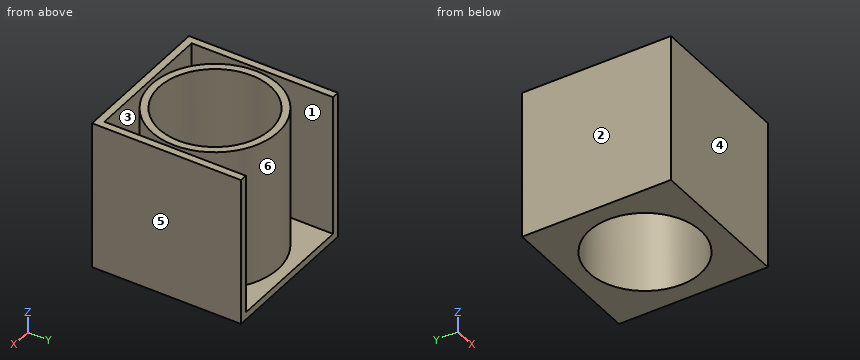
```python
from build123d import *

# Parameters (mm, degrees)
F0_W     = 50
F0_H     = 50
F1_DEPTH = 50
F2_R     = 18.7425
F3_DEPTH = 50
F4_T     = -2.5


with BuildPart() as f1:
    # F0 (on Top) → F1 (new body)
    with BuildSketch(Plane.XY):
        Rectangle(F0_W, F0_H)
    extrude(amount=F1_DEPTH)

    # F2 (on face) → F3 (cut)
    with BuildSketch(Plane.XY.offset(50)):
        Circle(F2_R)
    extrude(amount=-F3_DEPTH, mode=Mode.SUBTRACT)

    # F4
    f4_openings = [f1.faces().sort_by_distance(p)[0] for p in [
        (24.292893, 0, 50),
        (0, 25, 25),
    ]]
    offset(amount=F4_T, openings=f4_openings)


solid = f1.part
```
Verification items for the finished model (mm, model axes). Face numbers are marked on the shaded views. A direction names the side the tool comes from. Round coordinates to 2 decimals unless told otherwise and drop trailing zeros. Write each loop counter-clockwise with the first axis right and the second up, starting at its lowest first coordinate (ties: lowest second). Pieces come first, ordered by that corner, then holes. Notation, with made-up numbers: (-15.5, 25) - (43.5, 25) arc R14 ccw to (43.5, 48) - close; hole circle Ø4 at (25.25, -19). An arc over 180 degrees is marked (long way). Answer as a JSON object with one key per item and string values. Group by question number.
Q1. Thickness scan on line 1 (Y direction, x = 0, z = 13); line 2 (X direction, y = 22.5, z = 31); line 3 (Y direction, x = -17, z = 24). Record the ranges inside material, lowest first.
Q2. Section check D-D, the plane x = 7.5. Enter the section's corners in (y, z).
Q3. Section check C-C, the plane x = 0. Enter the section's corners in (y, z), plus the area to 3 significant figures.
Q4. Mould release check, pull along X, two halves, no side actions. Record for the marked faces 4, 5 and 6: released by +X, released by -X, zero draft, split by the parting line, or undercut.
Q5. Section check B-B, the plane y = 0. Enter the section's corners in (x, z).
Q6. Section check A-A, the plane z = 29.5. Enter the section's corners in (x, y) (1 decimal).
Q7. Go/stop test with flat-tipped pins: pin 1 Ø4 at (x, z) = (16.5, 7) entering from +Y; pin 2 Ø8 at (x, z) = (-4, 35.5) entering from +Y; pin 3 Ø3 at (x, z) = (-15.5, 9) entering from +Y. Record where each tip stops, or that it passes through.
Q8. Tool access check on the marked faces 1, 2 and 3. Record the directions out of +Z, -Z, +X, -X, +Y, -Y that give a thin tool (end or side, any length) a straight path to the whole face; none if there is none.
Found:
{
 "1": {"line 1": "y = -25 to -22.5, -21.24 to -18.74, 18.74 to 21.24", "line 2": "x = -25 to -22.5, 22.5 to 25", "line 3": "y = -25 to -22.5, -12.74 to -7.89, 7.89 to 12.74"},
 "2": {"outline": "(-25, 0) - (-17.18, 0) - (-17.18, 50) - (-19.87, 50) - (-19.87, 2.5) - (-22.5, 2.5) - (-22.5, 50) - (-25, 50) - close; (17.18, 0) - (25, 0) - (25, 2.5) - (19.87, 2.5) - (19.87, 50) - (17.18, 50) - close"},
 "3": {"outline": "(-25, 0) - (-18.74, 0) - (-18.74, 50) - (-21.24, 50) - (-21.24, 2.5) - (-22.5, 2.5) - (-22.5, 50) - (-25, 50) - close; (18.74, 0) - (25, 0) - (25, 2.5) - (21.24, 2.5) - (21.24, 50) - (18.74, 50) - close", "area": "388 mm^2"},
 "4": {"face 4": "zero draft", "face 5": "released by +X", "face 6": "undercut"},
 "5": {"outline": "(-25, 0) - (-18.74, 0) - (-18.74, 50) - (-21.24, 50) - (-21.24, 2.5) - (-22.5, 2.5) - (-22.5, 50) - (-25, 50) - close; (18.74, 0) - (25, 0) - (25, 50) - (22.5, 50) - (22.5, 2.5) - (21.24, 2.5) - (21.24, 50) - (18.74, 50) - close"},
 "6": {"outline": "(-25, -25) - (25, -25) - (25, 25) - (22.5, 25) - (22.5, -22.5) - (-22.5, -22.5) - (-22.5, 25) - (-25, 25) - close; circle Ø42.5 at (0, 0); hole circle Ø37.5 at (0, 0)"},
 "7": {"pin 1": "stops at y = 15.52", "pin 2": "stops at y = 21.24", "pin 3": "stops at y = 15.98"},
 "8": {"face 1": "+Z, +Y", "face 2": "+Z, -Z, -X, +Y, -Y", "face 3": "+Z"}
}
